Check sheet for the drawn part. Datum: minimum x, y, z corner. Units: mm. Round coordinates to 2 decimals unless told otherwise and drop trailing zeros. Write each loop counter-clockwise with the first axis right and the second up, starting at its lowest first coordinate (ties: lowest second). Pieces come first, ordered by that corner, then holes. Notation, with made-up numbers: M 89.5,75.25 L 122.5,75.25 A13 ccw 122.5,90.25 Z; hole C 52,-7 d1. An arc over 180 degrees is marked long. One line per item, written item: value. Start each with the question number.
Item 1: Section check D-D, the plane y = 10.75. Record the cut outline in (x, z), then the cut area to 3 significant figures.
Item 2: Gauge pin test, flat ends, axial feed: pin 1 (2.5 mm diameter, centred on x = 3, y = 10.5, fed in from -Z); pin 2 (1.5 mm diameter, centred on x = 0.5, z = 4, fed in from +Y); pin 3 (1.8 mm diameter, centred on x = 2.45, z = 2.45, fed in from -Y). Record the tip position at first contact, or that the pin passes through.
Item 3: Draft check along X on the marked faces 1, 2, 3 and 4. Enter one of: +X half, -X half, draft (parallel to the pull), parting line (faces both ways), or undercut.
Item 4: Section check A-A, the plane z = 2.45. Record the cut outline in (x, y), then the cut area to 4 significant figures.
Item 5: Section check C-C, the plane z = 3.3. Record the cut outline in (x, y).
Item 6: Section check B-B, the plane x = 2.45. Record the cut outline in (y, z), then the cut area to 3 significant figures.
Item 7: Thickness scan on probe 1 along Z at (x, y) = (2.45, 6); probe 2 along X at (y, z) = (7.5, 2.4); probe 3 along Z at (x, y) = (2.45, 9.75). Record the ranges inside material, lowest first. Write a range as from..to.
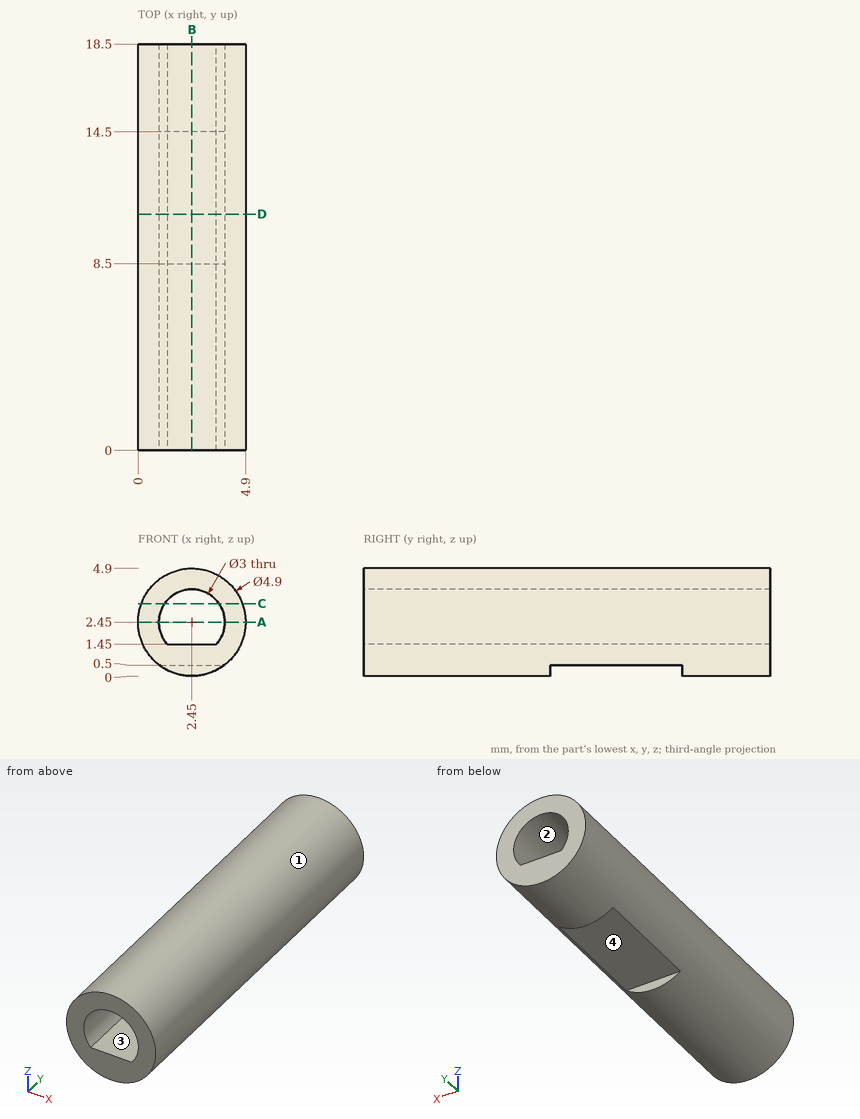
Response values:
1. outline: M 0.97,0.5 L 3.93,0.5 A2.45 ccw long Z; hole M 1.33,1.45 L 3.57,1.45 A1.5 ccw long Z
1. area: 11.6 mm2
2. pin 1: stops at z = 0.5
2. pin 2: stops at y = 18.5
2. pin 3: passes through
3. face 1: parting line
3. face 2: undercut
3. face 3: undercut
3. face 4: draft
4. outline: M 0,0 L 0.95,0 L 0.95,18.5 L 0,18.5 Z; M 3.95,0 L 4.9,0 L 4.9,18.5 L 3.95,18.5 Z
4. area: 35.15 mm2
5. outline: M 0.15,0 L 1.21,0 L 1.21,18.5 L 0.15,18.5 Z; M 3.69,0 L 4.75,0 L 4.75,18.5 L 3.69,18.5 Z
6. outline: M 0,0 L 8.5,0 L 8.5,0.5 L 14.5,0.5 L 14.5,0 L 18.5,0 L 18.5,1.45 L 0,1.45 Z; M 0,3.95 L 18.5,3.95 L 18.5,4.9 L 0,4.9 Z
6. area: 41.4 mm2
7. probe 1: z = 0..1.45, 3.95..4.9
7. probe 2: x = 0..0.95, 3.95..4.9
7. probe 3: z = 0.5..1.45, 3.95..4.9
